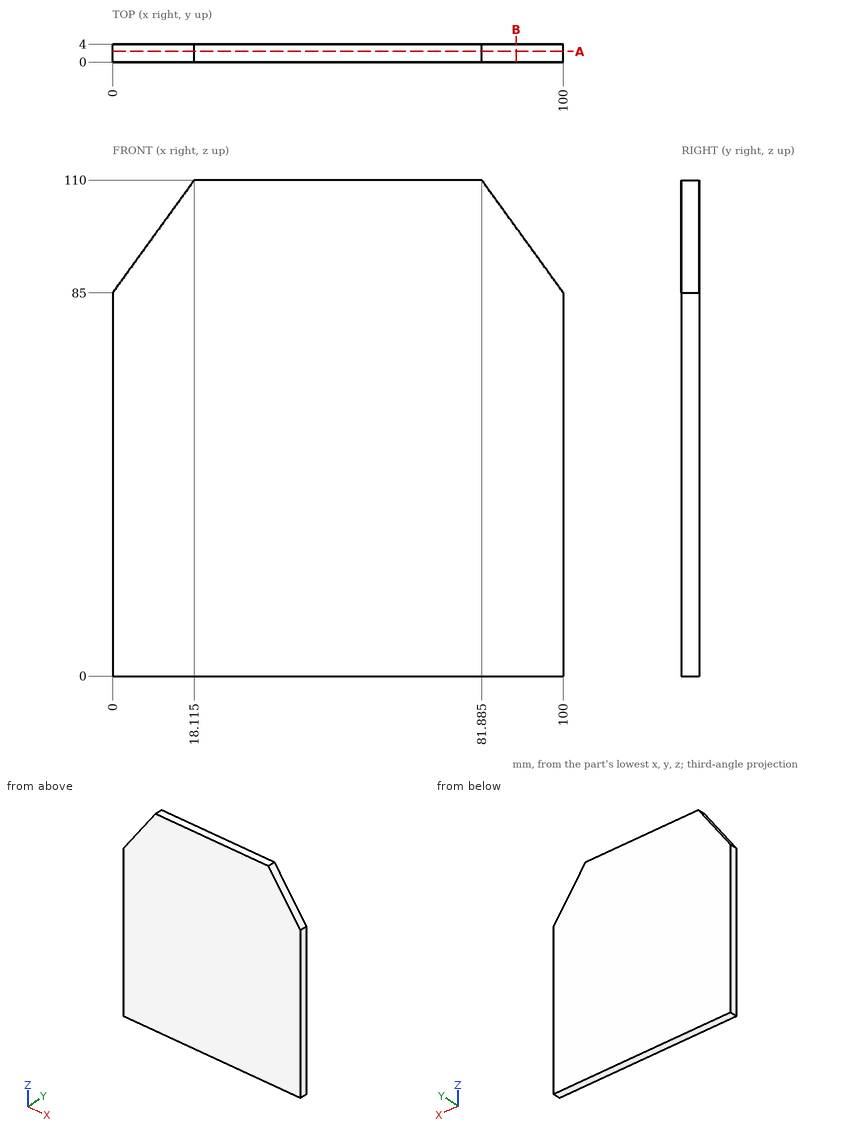
Part print with two shaded views. Sizes in mm from the minimum x, y, z corner. Coordinates: 2 decimals unless noted, no trailing zeros. Write each loop counter-clockwise with the first axis right and the second up, starting at its lowest first coordinate (ties: lowest second). Pieces come first, ordered by that corner, then holes.
1. Band-saw the part on B-B, the plane x = 89.5. Give the cut face in (y, z), and give its area (3 significant figures).
Answer block:
outline: (0, 0) - (4, 0) - (4, 99.49) - (0, 99.49) - close
area: 398 mm2
2. Band-saw the part on A-A, the plane y = 2.35. Give the cut face in (x, z) (3 decimals), and give its area (3 significant figures).
Answer block:
outline: (0, 0) - (100, 0) - (100, 85) - (81.885, 110) - (18.115, 110) - (0, 85) - close
area: 10,500 mm2
3. Drill centre lines: probe 1 along Z at (x, y) = (95, 0.2); probe 2 along X at (y, z) = (0.35, 100); probe 3 along Z at (x, y) = (84.5, 2.1). Where is each one in solid material? Low to high.
Answer block:
probe 1: z = 0 to 91.9
probe 2: x = 10.87 to 89.13
probe 3: z = 0 to 106.39
